Job drawing, mm, ordinate dimensions from the low corner. One solid piece. A direction names the side the tool comes from. Give positions to 0.01 mm unless a question says otherwise; leave off trailing zeros. Order: outer loops, then holes, each group sorted by start corner. A loop starts at its lowest first (then second) coordinate and runs counter-clockwise, first axis right, second up.
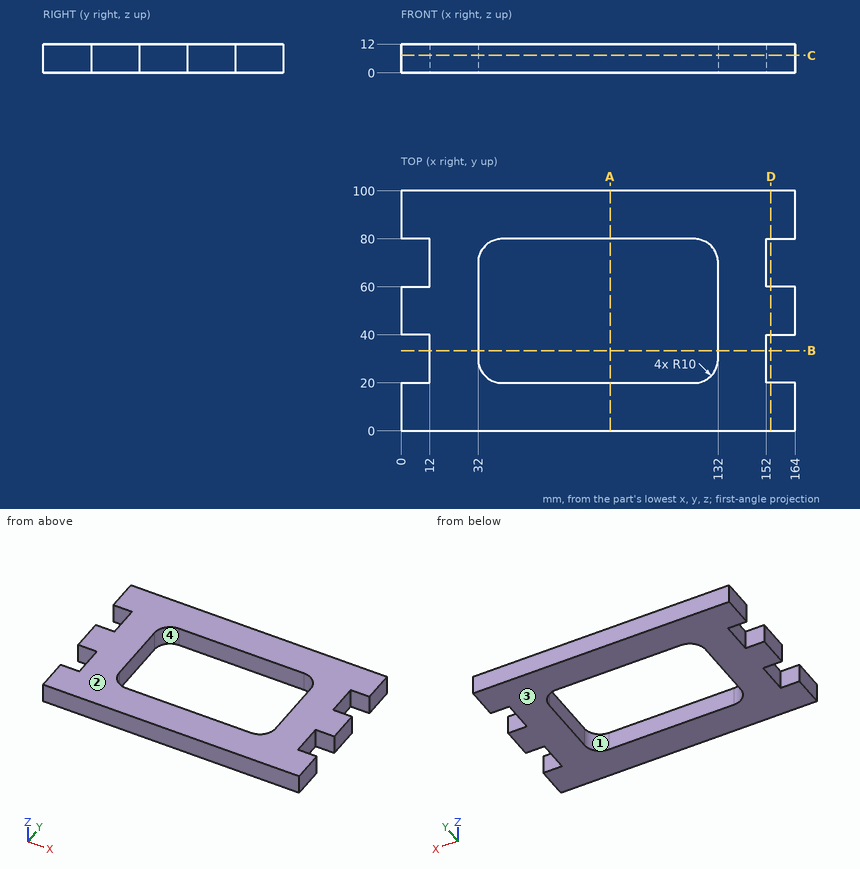
Item 1: Which spindle directions (+Z, -Z, +X, -X, +Y, -Y) get a long thin tool onto all of the face, cutting with end or side? Do the marked faces 3 and 4. Say none if no direction does.
Item 2: Band-saw the part on A-A on x = 87. List the corners of the cut face in (y, z), plus the area to 3 significant figures.
Item 3: Band-saw the part on B-B on y = 33.5. List the corners of the cut face in (x, z), plus the area to 3 significant figures.
Item 4: Drop flat-ended pins along their axis: P1, Ø1.5, axis at y = 66.5, z = 4.5, coming from the -X side; P2, Ø1.5, axis at y = 22, z = 2.5, coming from the +X side. Give the stop position or say it passes through.
Item 5: Band-saw the part on D-D on x = 154. List the corners of the cut face in (y, z), plus the area to 3 significant figures.
Item 6: Drill centre lines: probe 1 along X at (y, z) = (33.5, 5.25); probe 2 along Y at (x, z) = (48, 10.25); probe 3 along X at (y, z) = (52.5, 11.75). Where is each one in solid material? Low to high.
Item 7: Pull direction Y, two halves, no side cores. Call the marked faces 1 and 2: released by +Y, released by -Y, zero draft, split by the parting line, or undercut.
Item 8: Band-saw the part on C-C on z = 7.25. List the corners of the cut face in (x, y), plus the area to 3 significant figures.
Working result:
1. face 3: -Z, +X, -X, +Y, -Y
1. face 4: +Z, -Z
2. outline: (0, 0) - (20, 0) - (20, 12) - (0, 12) - close; (80, 0) - (100, 0) - (100, 12) - (80, 12) - close
2. area: 480 mm2
3. outline: (12, 0) - (32, 0) - (32, 12) - (12, 12) - close; (132, 0) - (152, 0) - (152, 12) - (132, 12) - close
3. area: 480 mm2
4. P1: stops at x = 12
4. P2: stops at x = 152
5. outline: (0, 0) - (20, 0) - (20, 12) - (0, 12) - close; (40, 0) - (60, 0) - (60, 12) - (40, 12) - close; (80, 0) - (100, 0) - (100, 12) - (80, 12) - close
5. area: 720 mm2
6. probe 1: x = 12 to 32, 132 to 152
6. probe 2: y = 0 to 20, 80 to 100
6. probe 3: x = 0 to 32, 132 to 164
7. face 1: undercut
7. face 2: zero draft
8. outline: (0, 0) - (164, 0) - (164, 20) - (152, 20) - (152, 40) - (164, 40) - (164, 60) - (152, 60) - (152, 80) - (164, 80) - (164, 100) - (0, 100) - (0, 80) - (12, 80) - (12, 60) - (0, 60) - (0, 40) - (12, 40) - (12, 20) - (0, 20) - close; hole (32, 30) arc R10 ccw to (42, 20) - (122, 20) arc R10 ccw to (132, 30) - (132, 70) arc R10 ccw to (122, 80) - (42, 80) arc R10 ccw to (32, 70) - close
8. area: 9,530 mm2
